Geometry: final body of the model. Coordinates: model frame, mm. A direction names the side the tool comes from. Round coordinates to 2 decimals unless told otherwise and drop trailing zeros. Loops run counter-clockwise (first coordinate to the right, second up) from the corner with the lowest first, then second, coordinate; pieces in that order, holes last. Notation, with made-up numbers: M 36,-6 L 41,-6 A12 ccw 41,2 Z; hole C -37,60.25 d7. An arc over 180 degrees is marked long. Answer as a JSON object with one key per item and string values.
```python
from build123d import *

# Parameters (mm, degrees)
SKETCH_W     = 5.867174
SKETCH_H     = 0.6
POCKET_DEPTH = 0.5


with BuildPart() as part:
    # Sketch001 → Revolution (revolve)
    with BuildSketch(Plane.XZ):
        Polygon((0, 0), (1.5, 0), (1.5, 11.8), (2.75, 11.8), (2.75, 13.9), (0, 13.9), align=None)
    revolve(axis=Axis((0, 0, 0), (0, 0, 1)))

    # Sketch → Pocket (cut)
    with BuildSketch(Plane(origin=(0, 0, 13.9), x_dir=(-1, 0, 0), z_dir=(0, 0, 1))):
        Rectangle(SKETCH_W, SKETCH_H)
    extrude(amount=-POCKET_DEPTH, mode=Mode.SUBTRACT)


solid = part.part
```
1) Cut plane C-C on z = 13.25. Return the cut outline in (x, y).
Geometry results:
{"outline": "C 0,0 d5.5"}
2) Cut plane D-D on y = 0.6. Return the cut outline in (x, z), and give its area (3 significant figures).
Geometry results:
{"outline": "M -2.68,11.8 L -1.37,11.8 L -1.37,0 L 1.37,0 L 1.37,11.8 L 2.68,11.8 L 2.68,13.9 L -2.68,13.9 Z", "area": "43.7 mm2"}
3) Cut plane A-A on y = 0. Return the cut outline in (x, z), and give its area (3 significant figures).
Geometry results:
{"outline": "M -2.75,11.8 L -1.5,11.8 L -1.5,0 L 1.5,0 L 1.5,11.8 L 2.75,11.8 L 2.75,13.4 L -2.75,13.4 Z", "area": "44.2 mm2"}
4) Cut plane B-B on x = 0. Return the cut outline in (y, z).
Geometry results:
{"outline": "M -2.75,11.8 L -1.5,11.8 L -1.5,0 L 1.5,0 L 1.5,11.8 L 2.75,11.8 L 2.75,13.9 L 0.3,13.9 L 0.3,13.4 L -0.3,13.4 L -0.3,13.9 L -2.75,13.9 Z"}
5) Line query: probe 1 along X at (y, z) = (-0.1, 6.25); probe 2 along Z at (x, y) = (-1.8, -1.6); probe 3 along Z at (x, y) = (0.3, -0.15). Output: solid intervals per line, ascending.
Geometry results:
{"probe 1": "-1.5 to 1.5", "probe 2": "11.8 to 13.9", "probe 3": "0 to 13.4"}
6) Set-up query: faces 1 (the face through (-1.2, -1.2, 11.8)), 2 (the face through (0, 1, 13.9)). Return all of +Z, -Z, +X, -X, +Y, -Y with unobstructed straight access to the full face (end or side cutting, diameter ignored); none if empty.
Geometry results:
{"face 1": "-Z", "face 2": "+Z, +X, -X, +Y, -Y"}
7) First-contact query: pin 1 (0.5 mm diameter, centred on x = 0.5, y = 0, fed in from +Z); pin 2 (3 mm diameter, centred on y = -0.5, z = 2, fed in from -X); pin 3 (1.5 mm diameter, centred on x = 2, y = 2, fed in from -Z). Flat tips, straight axial feed; report the tip coordinate or a pass-through.
Geometry results:
{"pin 1": "z = 13.4", "pin 2": "x = -1.5", "pin 3": "z = 11.8"}
